Input: dimensioned drawing with shaded views. Units: mm. Origin: part minimum x, y, z. Give positions to 0.01 mm unless a question says otherwise; leave off trailing zeros. Order: outer loops, then holes, each group sorted by start corner. A loop starts at its lowest first (then second) coordinate and runs counter-clockwise, first axis right, second up.
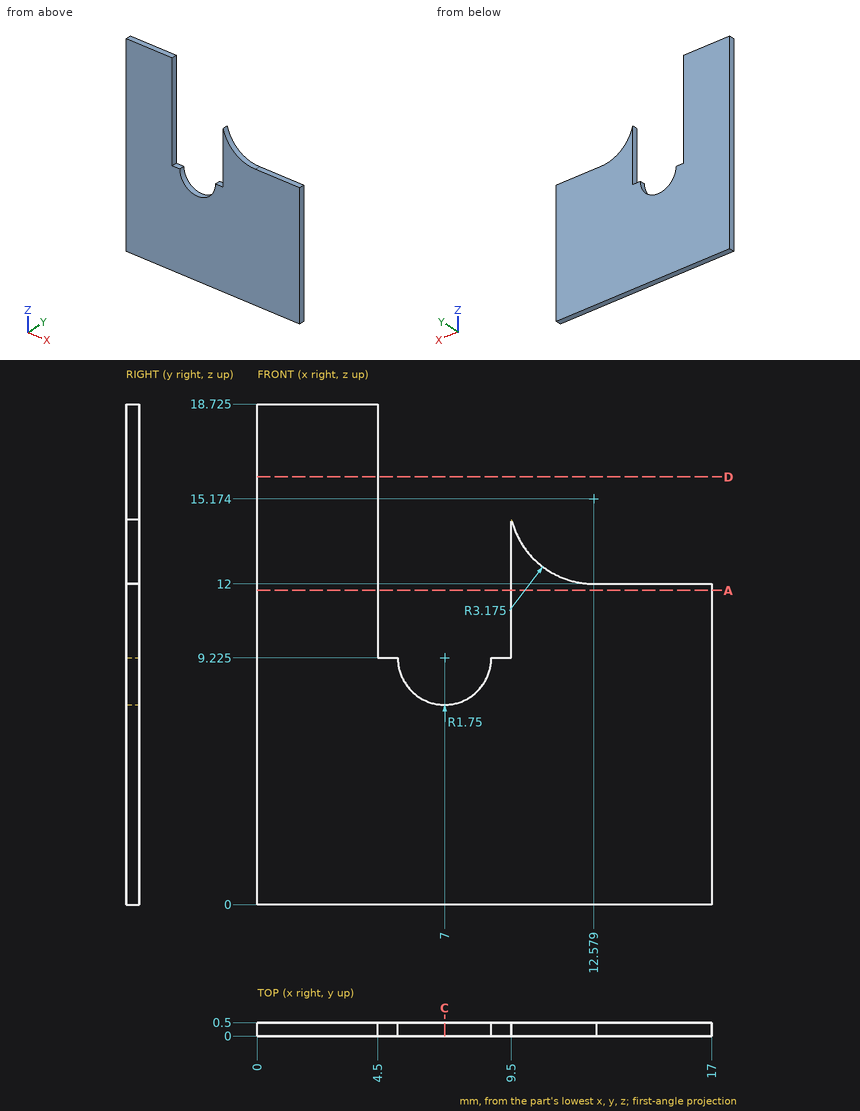
1) Section query D-D, the plane z = 16. Return the cut outline in (x, y).
Report:
outline: (0, 0) - (4.5, 0) - (4.5, 0.5) - (0, 0.5) - close
2) Section query A-A, the plane z = 11.75. Return the cut outline in (x, y).
Report:
outline: (0, 0) - (4.5, 0) - (4.5, 0.5) - (0, 0.5) - close; (9.5, 0) - (17, 0) - (17, 0.5) - (9.5, 0.5) - close
3) Pin query (flat end, axial travel): pin 1 (2 mm diameter, centred on x = 10, z = 10, fed in from -Y). Return the tip coordinate at first contact, or that it passes through.
Report:
pin 1: stops at y = 0
4) Material intervals for L1, parallel to X at y = 0.2, z = 16.5; L2, parallel to Z at x = 16.75, y = 0.1; L3, parallel to Z at x = 5, y = 0.2 (1 decimal), sorted ascending.
Report:
L1: x = 0 to 4.5
L2: z = 0 to 12
L3: z = 0 to 9.2
5) Section query C-C, the plane x = 7. Return the cut outline in (y, z) (1 decimal).
Report:
outline: (0, 0) - (0.5, 0) - (0.5, 7.5) - (0, 7.5) - close
